Build history of the part. All positions in model axes, mm. Face numbers are marked on the shaded views. A direction names the side the tool comes from. Round coordinates to 2 decimals unless told otherwise and drop trailing zeros. Write each loop counter-clockwise with the first axis right and the second up, starting at its lowest first coordinate (ties: lowest second). Pieces come first, ordered by that corner, then holes. Notation, with made-up numbers: (-3.75, 76.5) -> (8.25, 76.5) arc R20 cw to (8.25, 92.5) -> close; hole circle Ø3 at (47, -19). An arc over 180 degrees is marked (long way). Answer in a Markdown table with one row per item. Add a question column.
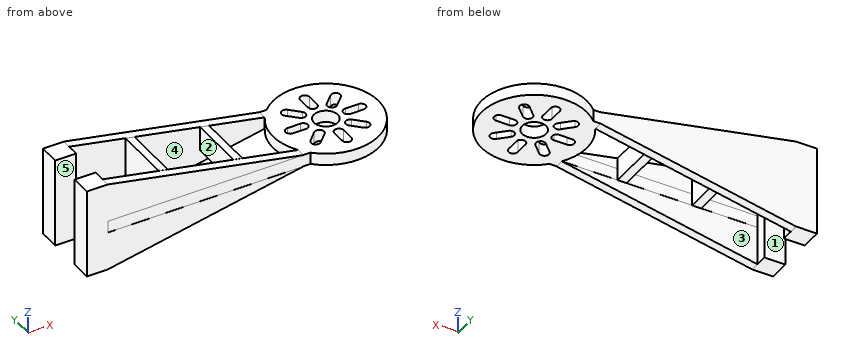
from build123d import *

# Parameters (mm, degrees)
SKETCH_1_R      = 4
EXTRUDE_3_DEPTH = 4
EXTRUDE_5_DEPTH = 3
EXTRUDE_6_DEPTH = 3
SKETCH_7_W      = 29.9977514
SKETCH_7_H      = 6.971398352
EXTRUDE_7_DEPTH = 7
EXTRUDE_8_DEPTH = 19
EXTRUDE_9_DEPTH = 19


with BuildPart() as part:
    # 草图1 → 凸台-拉伸3 (new body)
    with BuildSketch(Plane.XY):
        with BuildLine():
            Line((-39.928997061, 12.519020092), (-39.928997061, 9.519020095))
            Line((-39.928997061, 9.519020095), (25.662951423, 9.519020095))
            ThreePointArc((25.662951423, 9.519020095), (22.825216093, 0.019020096), (25.662951419, -9.480979905))
            Line((25.662951419, -9.480979905), (-39.928997061, -9.480979905))
            Line((-39.928997061, -9.480979905), (-39.928997061, -12.480979908))
            Line((-39.928997061, -12.480979908), (28.071002939, -12.480979908))
            ThreePointArc((28.071002939, -12.480979908), (58.248672468, 0.019020092), (28.071002939, 12.519020092))
            Line((28.071002939, 12.519020092), (-39.928997061, 12.519020092))
        make_face()
        with Locations((40.571002939, 0.019020092)):
            Circle(SKETCH_1_R, mode=Mode.SUBTRACT)
        with BuildLine():
            Line((28.614427542, 1.55), (33.014427542, 1.55))
            ThreePointArc((33.014427542, 1.55), (34.564427542, 0), (33.014427542, -1.55))
            Line((33.014427542, -1.55), (28.614427542, -1.55))
            ThreePointArc((28.614427542, -1.55), (27.064427542, 0), (28.614427542, 1.55))
        make_face(mode=Mode.SUBTRACT)
        with BuildLine():
            Line((52.385572458, 1.55), (47.985572458, 1.55))
            ThreePointArc((47.985572458, 1.55), (46.435572458, 0), (47.985572458, -1.55))
            Line((47.985572458, -1.55), (52.385572458, -1.55))
            ThreePointArc((52.385572458, -1.55), (53.935572458, 0), (52.385572458, 1.55))
        make_face(mode=Mode.SUBTRACT)
        with BuildLine():
            Line((42.101982847, -11.937555304), (42.101982847, -7.537555304))
            ThreePointArc((42.101982847, -7.537555304), (40.551982847, -5.987555304), (39.001982847, -7.537555304))
            Line((39.001982847, -7.537555304), (39.001982847, -11.937555304))
            ThreePointArc((39.001982847, -11.937555304), (40.551982847, -13.487555304), (42.101982847, -11.937555304))
        make_face(mode=Mode.SUBTRACT)
        with BuildLine():
            Line((33.29940699, 9.45574859), (36.410676827, 6.344478753))
            ThreePointArc((36.410676827, 6.344478753), (36.410676827, 4.152447732), (34.218645805, 4.152447732))
            Line((34.218645805, 4.152447732), (31.107375968, 7.263717569))
            ThreePointArc((31.107375968, 7.263717569), (31.107375968, 9.45574859), (33.29940699, 9.45574859))
        make_face(mode=Mode.SUBTRACT)
        with BuildLine():
            Line((42.05, 11.885572458), (42.05, 7.485572458))
            ThreePointArc((42.05, 7.485572458), (40.5, 5.935572458), (38.95, 7.485572458))
            Line((38.95, 7.485572458), (38.95, 11.885572458))
            ThreePointArc((38.95, 11.885572458), (40.5, 13.435572458), (42.05, 11.885572458))
        make_face(mode=Mode.SUBTRACT)
        with BuildLine():
            Line((47.70059301, 9.45574859), (44.589323173, 6.344478753))
            ThreePointArc((44.589323173, 6.344478753), (44.589323173, 4.152447732), (46.781354195, 4.152447732))
            Line((46.781354195, 4.152447732), (49.892624032, 7.263717569))
            ThreePointArc((49.892624032, 7.263717569), (49.892624032, 9.45574859), (47.70059301, 9.45574859))
        make_face(mode=Mode.SUBTRACT)
        with BuildLine():
            Line((33.29940699, -9.45574859), (36.410676827, -6.344478753))
            ThreePointArc((36.410676827, -6.344478753), (36.410676827, -4.152447732), (34.218645805, -4.152447732))
            Line((34.218645805, -4.152447732), (31.107375968, -7.263717569))
            ThreePointArc((31.107375968, -7.263717569), (31.107375968, -9.45574859), (33.29940699, -9.45574859))
        make_face(mode=Mode.SUBTRACT)
        with BuildLine():
            Line((47.70059301, -9.45574859), (44.589323173, -6.344478753))
            ThreePointArc((44.589323173, -6.344478753), (44.589323173, -4.152447732), (46.781354195, -4.152447732))
            Line((46.781354195, -4.152447732), (49.892624032, -7.263717569))
            ThreePointArc((49.892624032, -7.263717569), (49.892624032, -9.45574859), (47.70059301, -9.45574859))
        make_face(mode=Mode.SUBTRACT)
    extrude(amount=EXTRUDE_3_DEPTH)

    # 草图2 → 凸台-拉伸5 (add)
    with BuildSketch(Plane(origin=(0, 12.519020092, 0), x_dir=(1, 0, 0), z_dir=(0, 1, 0))):
        Polygon((-39.928997061, 0), (-39.928997061, 13), (25.661002939, 0), align=None)
    extrude_5 = extrude(amount=-EXTRUDE_5_DEPTH)

    # 镜向1: 凸台-拉伸5 across plane
    add(extrude_5.mirror(Plane.ZX))

    # 草图5 → 凸台-拉伸6 (add)
    with BuildSketch(Plane(origin=(0, 12.519020092, 0), x_dir=(1, 0, 0), z_dir=(0, 1, 0))):
        Polygon((-39.928997061, -4), (-39.928997061, -17), (25.661002939, -4), align=None)
    extrude_6 = extrude(amount=-EXTRUDE_6_DEPTH)

    # 镜向2: 凸台-拉伸6 across plane
    add(extrude_6.mirror(Plane.ZX))

    # 草图7 → 凸台-拉伸7 (add)
    with BuildSketch(Plane.ZY.offset(39.928997061)):
        with Locations((1.9988757, 9.033320916)):
            Rectangle(SKETCH_7_W, SKETCH_7_H)
    extrude_7 = extrude(amount=EXTRUDE_7_DEPTH)

    # 镜向3: 凸台-拉伸7 across plane
    add(extrude_7.mirror(Plane.ZX))

    # 草图8 → 凸台-拉伸8 (add)
    with BuildSketch(Plane.XZ.offset(-9.519020095)):
        Polygon((-21.039670639, 0), (-18.039670639, 0), (-18.039670639, 12.661514812), (-21.039670639, 13.256117648), align=None)
    extrude(amount=EXTRUDE_8_DEPTH)

    # 草图9 → 凸台-拉伸9 (add)
    with BuildSketch(Plane.XZ.offset(-9.519020095)):
        Polygon((4, 0), (7, 0), (7, 7.698628422), (4, 8.293231258), align=None)
    extrude(amount=EXTRUDE_9_DEPTH)


solid = part.part
(1) Saw through at A-A (z = -2.75). List the corners of the cut face in (x, y).
(2) Which spindle directions (+Z, -Z, +X, -X, +Y, -Y) get a long thin tool onto all of the face, cutting with end or side? Do the marked faces 1, 2 and 3. Say none if no direction does.
(3) Mould opens along X. For the marked faces 4 and 5 say: pulls with the +X half, pulls with the -X half, needs draft (parallel to the pull), parting line crosses it, or undercut.
(4) Probe line 1 along Y through (x, z) = (-0.5, 6.25); line 2 along Z through (x, y) = (48, -11); line 3 along X through (y, z) = (6, -8.75). List the from-to ranges inside material, lowest first.
(5) Saw through at D-D (z = -9.25). List the corners of the cut face in (x, y), plus the area to 3 significant figures.
(6) Saw through at C-C (x = 40.5). List the corners of the cut face in (y, z), plus the area to 3 significant figures.
(7) Drop flat-ended pins along their axis: P1, Ø2, axis at x = 32, z = 3, coming from the -Y side; P2, Ø3, axis at x = 30.5, z = 2, coming from the +Y side; P3, Ø5, axis at y = 3.5, z = 12.5, coming from the +X side; P4, Ø1, axis at x = 22.5, y = -14, coming from the -Z side. Give the stop position or say it passes through.
Answer sheet:
| question | item | result |
|---|---|---|
| 1 | outline | (-46.93, -12.52) -> (11.79, -12.52) -> (11.79, -9.52) -> (-39.93, -9.52) -> (-39.93, -5.55) -> (-46.93, -5.55) -> close; (-46.93, 5.55) -> (-39.93, 5.55) -> (-39.93, 9.52) -> (11.79, 9.52) -> (11.79, 12.52) -> (-46.93, 12.52) -> close |
| 2 | face 1 | +Z, -Z, -X |
| 2 | face 2 | +Z, -Z |
| 2 | face 3 | -Z, +X |
| 3 | face 4 | undercut |
| 3 | face 5 | needs draft |
| 4 | line 1 | y = -12.52 to -9.52, 9.52 to 12.52 |
| 4 | line 2 | z = 0 to 4 |
| 4 | line 3 | x = -46.93 to -39.93 |
| 5 | outline | (-46.93, -12.52) -> (-21.01, -12.52) -> (-21.01, -9.52) -> (-39.93, -9.52) -> (-39.93, -5.55) -> (-46.93, -5.55) -> close; (-46.93, 5.55) -> (-39.93, 5.55) -> (-39.93, 9.52) -> (-21.01, 9.52) -> (-21.01, 12.52) -> (-46.93, 12.52) -> close |
| 5 | area | 211 mm² |
| 6 | outline | (-17.66, 0) -> (-13.49, 0) -> (-13.49, 4) -> (-17.66, 4) -> close; (-5.99, 0) -> (-3.98, 0) -> (-3.98, 4) -> (-5.99, 4) -> close; (4.02, 0) -> (5.94, 0) -> (5.94, 4) -> (4.02, 4) -> close; (13.44, 0) -> (17.7, 0) -> (17.7, 4) -> (13.44, 4) -> close |
| 6 | area | 49.4 mm² |
| 7 | P1 | stops at y = -15.96 |
| 7 | P2 | stops at y = 15.48 |
| 7 | P3 | stops at x = -18.04 |
| 7 | P4 | passes through |
